CAD build for the part. Positions are in the model's coordinates, mm. A direction names the side the tool comes from. Coordinates: 2 decimals unless noted, no trailing zeros. Order: outer loops, then holes, each group sorted by start corner. A loop starts at its lowest first (then second) coordinate and runs counter-clockwise, first axis right, second up. Notation, with made-up numbers: (26, 52.5) - (64, 52.5) arc R16 cw to (64, 73.5) - close; hole circle Ø6 at (-24, 55). An arc over 180 degrees is marked (long way). Use one line per item in the form item = value.
```python
from build123d import *

# Parameters (mm, degrees)
F0_W      = 25.4
F0_H      = 25.4
F1_DEPTH  = 25.4
F2_W      = 19.05
F2_H      = 19.05
F3_DEPTH  = 25.4
F4_W      = 19.05
F4_H      = 19.05
F5_DEPTH  = 25.4
F6_W      = 19.05
F6_H      = 19.05
F7_DEPTH  = 25.4
F9_DEPTH  = 3.175
F11_DEPTH = 3.175
F13_DEPTH = 3.175
F15_DEPTH = 3.175
F17_DEPTH = 3.175
F19_DEPTH = 3.175


with BuildPart() as f1:
    # F0 (on Front) → F1 (new body)
    with BuildSketch(Plane.XZ):
        with Locations((-4.7539575025, 3.3169323578)):
            Rectangle(F0_W, F0_H)
    extrude(amount=F1_DEPTH)

    # F2 (on face) → F3 (cut)
    with BuildSketch(Plane.XZ.offset(25.4)):
        with Locations((-4.7539575025, 3.3169323578)):
            Rectangle(F2_W, F2_H)
    extrude(amount=-F3_DEPTH, mode=Mode.SUBTRACT)

    # F4 (on face) → F5 (cut)
    with BuildSketch(Plane.YZ.offset(7.9460424975)):
        with Locations((-12.7, 3.3169323578)):
            Rectangle(F4_W, F4_H)
    extrude(amount=-F5_DEPTH, mode=Mode.SUBTRACT)

    # F6 (on face) → F7 (cut)
    with BuildSketch(Plane.XY.offset(16.0169323578)):
        with Locations((-4.7539575025, -12.7)):
            Rectangle(F6_W, F6_H)
    extrude(amount=-F7_DEPTH, mode=Mode.SUBTRACT)

    # F8 (on Front) → F9 (join)
    with BuildSketch(Plane.XZ):
        Polygon((7.9460424975, 3.3169323578), (-4.7539575025, 16.0169323578), (-17.4539575025, 3.3169323578), (-4.7539575025, -9.3830676422), align=None)
        Polygon((-14.2789575025, 3.3169323578), (-4.7539575025, 12.8419323578), (4.7710424975, 3.3169323578), (-4.7539575025, -6.2080676422), align=None, mode=Mode.SUBTRACT)
    extrude(amount=F9_DEPTH)

    # F10 (on face) → F11 (join)
    with BuildSketch(Plane.YZ.offset(7.9460424975)):
        Polygon((0, 3.3169323578), (-12.7, 16.0169323578), (-25.4, 3.3169323578), (-12.7, -9.3830676422), align=None)
        Polygon((-22.225, 3.3169323578), (-12.7, 12.8419323578), (-3.175, 3.3169323578), (-12.7, -6.2080676422), align=None, mode=Mode.SUBTRACT)
    extrude(amount=-F11_DEPTH)

    # F12 (on face) → F13 (join)
    with BuildSketch(Plane.XY.offset(16.0169323578)):
        Polygon((7.9460424975, -12.7), (-4.7539575025, 0), (-17.4539575025, -12.7), (-4.7539575025, -25.4), align=None)
        Polygon((-14.2789575025, -12.7), (-4.7539575025, -3.175), (4.7710424975, -12.7), (-4.7539575025, -22.225), align=None, mode=Mode.SUBTRACT)
    extrude(amount=-F13_DEPTH)

    # F14 (on face) → F15 (join)
    with BuildSketch(Plane(origin=(-17.4539575025, 0, 0), x_dir=(0, -1, 0), z_dir=(-1, 0, 0))):
        Polygon((25.4, 3.3169323578), (12.7, 16.0169323578), (0, 3.3169323578), (12.7, -9.3830676422), align=None)
        Polygon((3.175, 3.3169323578), (12.7, 12.8419323578), (22.225, 3.3169323578), (12.7, -6.2080676422), align=None, mode=Mode.SUBTRACT)
    extrude(amount=-F15_DEPTH)

    # F16 (on face) → F17 (join)
    with BuildSketch(Plane.XZ.offset(25.4)):
        Polygon((7.9460424975, 3.3169323578), (-4.7539575025, 16.0169323578), (-17.4539575025, 3.3169323578), (-4.7539575025, -9.3830676422), align=None)
        Polygon((-14.2789575025, 3.3169323578), (-4.7539575025, 12.8419323578), (4.7710424975, 3.3169323578), (-4.7539575025, -6.2080676422), align=None, mode=Mode.SUBTRACT)
    extrude(amount=-F17_DEPTH)

    # F18 (on face) → F19 (join)
    with BuildSketch(Plane(origin=(0, 0, -9.3830676422), x_dir=(1, 0, 0), z_dir=(0, 0, -1))):
        Polygon((7.9460424975, 12.7), (-4.7539575025, 25.4), (-17.4539575025, 12.7), (-4.7539575025, 0), align=None)
        Polygon((-14.2789575025, 12.7), (-4.7539575025, 22.225), (4.7710424975, 12.7), (-4.7539575025, 3.175), align=None, mode=Mode.SUBTRACT)
    extrude(amount=-F19_DEPTH)


solid = f1.part
```
Item 1: Drill centre lines: line 1 (Y direction, x = -7.75, z = 10) (3 decimals); line 2 (X direction, y = -16.25, z = -2.75); line 3 (X direction, y = -7.5, z = -8). Where is each one in solid material? Low to high. Write a range as [from, to].
Derived:
line_1 = [-25.4, -22.225], [-3.175, 0]
line_2 = [-17.45, -14.28], [4.77, 7.95]
line_3 = [-17.45, -14.28], [-12.25, -9.08], [-0.43, 2.75], [4.77, 7.95]
Item 2: Cut at A-A, the plane x = -6.5. Write the cut outline in (y, z) (3 decimals).
Derived:
outline = (-25.4, -9.383) - (-20.479, -9.383) - (-20.479, -6.208) - (-22.225, -6.208) - (-22.225, -4.462) - (-25.4, -4.462) - close; (-25.4, 11.096) - (-22.225, 11.096) - (-22.225, 12.842) - (-20.479, 12.842) - (-20.479, 16.017) - (-25.4, 16.017) - close; (-4.921, -9.383) - (0, -9.383) - (0, -4.462) - (-3.175, -4.462) - (-3.175, -6.208) - (-4.921, -6.208) - close; (-4.921, 12.842) - (-3.175, 12.842) - (-3.175, 11.096) - (0, 11.096) - (0, 16.017) - (-4.921, 16.017) - close
Item 3: Drop flat-ended pins along their axis: pin 1 (10 mm diameter, centred on x = 3.5, z = 4.5, fed in from +Y); pin 2 (8 mm diameter, centred on x = -6, z = 1, fed in from +Y). Give the stop position or say it passes through.
Derived:
pin_1 = 0
pin_2 = through
Item 4: Cut at D-D, the plane y = -19. State how many separate pieces and enclosed holes the cut face has, plus the area to 3 significant figures.
Derived:
separate_pieces = 12
enclosed_holes = 0
area = 121 mm²
Item 5: 3-axis set-ups, long thin cutter, end or side, ignore diameter. For faces 1 (the face through (1, -22.225, -2)), 2 (the face through (-11, -22.225, 14)), 3 (the face through (6, -22.225, -3)): which of +Z, -Z, +X, -X, +Y, -Y reach the whole face in a straight line?
Derived:
face_1 = none
face_2 = +Z, -Z
face_3 = +X, -X
Item 6: Cut at C-C, the plane y = -14.5. Write the cut outline in (x, z), plus the area to 3 significant figures.
Derived:
outline = (-17.45, -9.38) - (-12.48, -9.38) - (-12.48, -6.21) - (-14.28, -6.21) - (-14.28, -4.41) - (-17.45, -4.41) - close; (-17.45, 11.04) - (-14.28, 11.04) - (-14.28, 12.84) - (-12.48, 12.84) - (-12.48, 16.02) - (-17.45, 16.02) - close; (2.97, -9.38) - (7.95, -9.38) - (7.95, -4.41) - (4.77, -4.41) - (4.77, -6.21) - (2.97, -6.21) - close; (2.97, 12.84) - (4.77, 12.84) - (4.77, 11.04) - (7.95, 11.04) - (7.95, 16.02) - (2.97, 16.02) - close
area = 86.0 mm²
Item 7: Cut at B-B, the plane z = 14.5. Write the cut outline in (x, y) (3 decimals).
Derived:
outline = (-17.454, -25.4) - (7.946, -25.4) - (7.946, 0) - (-17.454, 0) - close; hole (-14.279, -22.225) - (-7.929, -22.225) - (-14.279, -15.875) - close; hole (-14.279, -12.7) - (-4.754, -22.225) - (4.771, -12.7) - (-4.754, -3.175) - close; hole (-14.279, -9.525) - (-7.929, -3.175) - (-14.279, -3.175) - close; hole (-1.579, -22.225) - (4.771, -22.225) - (4.771, -15.875) - close; hole (-1.579, -3.175) - (4.771, -9.525) - (4.771, -3.175) - close
Item 8: Two-plate mould, pull along X, no slides. Class faces 4 (the face through (2, -24, 12.842)), 5 (the face through (6.38, -17.53, 8.01)), 6 (the face through (-10, -3.175, -2)): +X half, -X half, draft (parallel to the pull), parting line (faces both ways), or undercut.
Derived:
face_4 = undercut
face_5 = draft
face_6 = undercut
